Geometry: final body of the model. Coordinates: model frame, mm. A direction names the side the tool comes from. Give positions to 0.01 mm unless a question says otherwise; leave off trailing zeros. Write each loop counter-clockwise with the first axis right and the second up, starting at its lowest first coordinate (ties: lowest second). Pieces come first, ordered by that corner, then holes. Notation, with made-up numbers: M 8,49 L 33,49 A32 ccw 33,85 Z; hole C -17,39.25 d2. An arc over 180 degrees is marked long. Use one line per item in the form item = value. Start each with the question number.
Item 1: Section query A-A on z = -45.5. Return loops of the section in (x, y).
Item 2: Section query B-B on z = 90. Return loops of the section in (x, y), then the cut area to 3 significant figures.
Item 3: Contact query for flat-ended pins moving along their axis: P1, Ø1, axis at x = 14, y = -5, coming from the -Z side; P2, Ø4, axis at y = 7.5, z = 28.5, coming from the +X side; P3, Ø2.5, axis at x = -8.5, z = 10, coming from the +Y side; P4, Ø1.5, axis at x = -5.5, y = -1, coming from the +Z side. Output: stop coordinate, or through.
Item 4: Section query C-C on x = 3.75. Return loops of the section in (y, z), then the cut area to 3 significant figures.
Item 5: Pull-direction query (X, two-part tool) for faces 5 (the flat face through (8, 5.85, -1)), 6 (the flat face through (-9.1, 3, -93)), 7 (the flat face through (11, -2, 1)); classes: released by +X, released by -X, zero draft, split by the parting line, or undercut.
Item 6: Material intervals for line 1 along Y through (x, z) = (-0.5, 90); line 2 along X through (y, z) = (0, -89.5); line 3 along X through (y, z) = (8, -82.5), sorted ascending. Write a range as from..to.
Item 7: Access query for faces 1 (the flat face through (-9.1, 3, 94)), 2 (the cylindrical face through (7.217, 10.962, -97.535)), 3 (the flat face through (9.1, 3, 94)), 4 (the cylindrical face through (8.34, 2.87, 80.55)). Directions: +Z, -Z, +X, -X, +Y, -Y. A direction counts if a zero-diameter tool reaches every point of the face in a straight line with its end or side. Return the directions, or none.
Autodesk Inventor part; units mm, degrees
ref_plane "YZ Plane" through (0, 0, 0) normal (1, 0, 0) x (0, 1, 0)
ref_plane "XZ Plane" through (0, 0, 0) normal (0, 1, 0) x (-1, 0, 0)
ref_plane "XY Plane" through (0, 0, 0) normal (0, 0, 1) x (1, 0, 0)
sketch "Sketch1" plane through (0, 0, 0) normal (0, 0, 1) x (1, 0, 0)
  line L0 (-11, -8.3) -> (11, -8.3)
  line L1 (11, -8.3) -> (11, 8.3)
  line L2 (11, 8.3) -> (-11, 8.3)
  line L3 (-11, 8.3) -> (-11, -8.3)
  line L4 (-11, -8.3) -> (11, 8.3) construction
  line L5 (11, -8.3) -> (-11, 8.3) construction
  line L6 (-5.6, 8.3) -> (-5.6, 5.8)
  line L7 (-5.6, 5.8) -> (-9.1, 5.8)
  line L8 (-9.1, 5.8) -> (-9.1, -0.2)
  line L9 (-9.1, -0.2) -> (-5.6, -0.2)
  line L10 (-5.6, -0.2) -> (-5.6, -3.2)
  line L11 (-5.6, -3.2) -> (0, -3.2)
  line L12 (0, 8.3) -> (0, -8.3) construction
  line L13 (5.6, 8.3) -> (5.6, 5.8)
  line L14 (5.6, 5.8) -> (9.1, 5.8)
  line L15 (9.1, 5.8) -> (9.1, -0.2)
  line L16 (9.1, -0.2) -> (5.6, -0.2)
  line L17 (5.6, -0.2) -> (5.6, -3.2)
  line L18 (5.6, -3.2) -> (0, -3.2)
  point P0 (0, 0)
  point P1 (-5.6, 7.05)
  point P2 (-5.6, -1.7)
  point P3 (5.6, 8.3)
  dimension "d0" = 22
  dimension "d1" = 16.6
  dimension "d3" = 5.6
  dimension "d4" = 2.5
  dimension "d5" = 6
  dimension "d6" = 3
  dimension "d7" = 3.5
  dimension "d36" = 18.2
extrude "Extrusion1" add sketch "Sketch1" along normal mid plane 200 contours L3 L2 L6 L7 L8 L9 L10 L11 L18 L17 L16 L15 L14 L13 L1 L0
sketch "Sketch2" plane through (11, -8.3, 100) normal (1, 0, 0) x (0, 0, -1)
  line L0 (200, 16.6) -> (200, 0)
  line L1 (200, 0) -> (0, 0)
  circle A0 centre (190, 3) radius 1.65
  line L2 (0, 0) -> (0, 16.6)
  line L3 (200, 16.6) -> (0, 16.6)
  line L4 (100, 16.6) -> (100, 0)
  circle A1 centre (10, 3) radius 1.65
  point P0 (100, 8.3)
  dimension "d13" = 3.3
  dimension "d18" = 180
  dimension "d19" = 3
extrude "Extrusion2" cut sketch "Sketch2" against normal blind 180 contours A0 | A1
sketch "Sketch5" plane through (-11, -8.3, 100) normal (-1, 0, 0) x (0, 0, 1)
  line L0 (-185, 11.1) -> (-15, 11.1) construction
  line L1 (-185, 8.05) -> (-15, 8.05)
  line L2 (-15, 14.15) -> (-185, 14.15)
  arc A0 (-185, 14.15) -> (-185, 8.05) centre (-185, 11.1) ccw
  arc A1 (-15, 8.05) -> (-15, 14.15) centre (-15, 11.1) ccw
  line L3 (-200, 14.1) -> (-200, 8.1)
  line L4 (-200, 0) -> (0, 0)
  line L5 (-200, 16.6) -> (0, 16.6)
  line L6 (-100, 16.6) -> (-100, 8.05)
  point P0 (-100, 8.3)
  point P1 (-100, 11.1)
  point P2 (-200, 11.1)
  point P3 (-100, 0)
  dimension "d23" = 85
  dimension "d24" = 6.1
extrude "Extrusion4" cut sketch "Sketch5" against normal up to next
sketch "Sketch6" plane through (0, 0, 100) normal (0, 0, 1) x (1, 0, 0)
  line L0 (-11, 8.3) -> (-5.6, 8.3)
  arc A0 (-6.6, 8.3) -> (-9.8, 9.9) centre (-8.6, 8.3) ccw
  line L1 (-5.6, 8.3) -> (-11, 8.3)
  arc A1 (-5.6, 8.3) -> (-10.4, 10.7) centre (-8.6, 8.3) ccw
  arc A2 (-10.4, 10.7) -> (-9.8, 9.9) centre (-10.1, 10.3) ccw
  line L2 (-11, 8.3) -> (-11, -8.3)
  point P0 (0, 0)
  point P1 (-6.5, 8.3)
  dimension "d29" = 2
  dimension "d31" = 1
  dimension "d32" = 2
extrude "Extrusion5" add sketch "Sketch6" against normal blind 5
mirror "Mirror1" about plane through (0, 0, 0) normal (1, 0, 0) of "Extrusion5"
mirror "Mirror2" about plane through (0, 0, 0) normal (0, 0, 1) of "Extrusion5", "Mirror1"
mirror "Mirror3" about plane through (0, 0, 0) normal (1, 0, 0) of "Extrusion4"
sketch "Sketch7" plane through (11, -8.3, 100) normal (1, 0, 0) x (0, 0, -1)
  line L0 (170, 11.1) -> (185, 11.1) construction
  line L1 (170, 8.05) -> (185, 8.05)
  line L2 (185, 14.15) -> (170, 14.15)
  arc A0 (170, 14.15) -> (170, 8.05) centre (170, 11.1) ccw
  arc A1 (185, 8.05) -> (185, 14.15) centre (185, 11.1) ccw
  arc A2 (185, 8.05) -> (185, 14.15) centre (185, 11.1) ccw
  arc A3 (177.5, 8.05) -> (177.5, 14.15) centre (177.5, 11.1) ccw
  point P0 (100, 8.3)
  dimension "d37" = 15
extrude "Extrusion6" add sketch "Sketch7" against normal up to surface (5.4 mm away) contours A3 L2 A1 L1
sketch "Sketch8" plane through (11, -8.3, 100) normal (1, 0, 0) x (0, 0, -1)
  circle A0 centre (182, 10.6) radius 0.95
  circle A1 centre (182, 3.6) radius 1.05
  line L0 (181.05, 4.0472) -> (181.05, 3.1528)
  line L1 (182, 4.65) -> (182, 2.55)
  line L2 (182.95, 4.0472) -> (182.95, 3.1528)
  line L3 (0, 16.6) -> (200, 16.6)
  line L4 (200, 16.6) -> (200, 0)
  point P0 (100, 8.3)
  point P1 (182.95, 3.1528)
  point P2 (182.95, 4.0472)
  dimension "d40" = 1.9
  dimension "d41" = 2.1
  dimension "d42" = 1.9
  dimension "d43" = 7
  dimension "d44" = 6
  dimension "d45" = 18
extrude "Extrusion7" add sketch "Sketch8" along normal blind 6.2 contours A0 | L2 A1 L1 | L1 A1 L0
mirror "Mirror4" about plane through (0, 0, 0) normal (0, 0, 1) of "Extrusion6", "Extrusion7"
ref_plane "Work Plane1" through (0, 0, 0) normal (1, 0, 0) x (0, 1, 0)
ref_plane "Work Plane2" through (0, 0, 0) normal (-1, 0, 0) x (0, 1, 0)
ref_plane "Work Plane3" through (0, 0, 0) normal (-1, 0, 0) x (0, 1, 0)
equation "\"d15\" = d18"
properties part number "Rack ( Female Fixation )"
Answer sheet:
q1.outline = M -11,-8.3 L 11,-8.3 L 11,-0.25 L 5.6,-0.25 L 5.6,-3.2 L -5.6,-3.2 L -5.6,-0.25 L -11,-0.25 Z; M -11,5.85 L -5.6,5.85 L -5.6,8.3 L -11,8.3 Z; M 5.6,5.85 L 11,5.85 L 11,8.3 L 5.6,8.3 Z
q2.outline = M -11,-8.3 L 11,-8.3 L 11,-6.95 L -11,-6.95 Z; M -11,-3.65 L 11,-3.65 L 11,8.3 L 5.6,8.3 L 5.6,5.8 L 9.1,5.8 L 9.1,-0.2 L 5.6,-0.2 L 5.6,-3.2 L -5.6,-3.2 L -5.6,-0.2 L -9.1,-0.2 L -9.1,5.8 L -5.6,5.8 L -5.6,8.3 L -11,8.3 Z
q2.area = 122 mm2
q3.P1 = -82.95
q3.P2 = 11
q3.P3 = 8.3
q3.P4 = 100
q4.outline = M -8.3,-100 L -3.2,-100 L -3.2,100 L -8.3,100 Z; hole C -5.3,-90 d3.3; hole C -5.3,90 d3.3
q4.area = 1,000 mm2
q5.face_5 = zero draft
q5.face_6 = undercut
q5.face_7 = released by +X
q6.line_1 = -8.3..-6.95, -3.65..-3.2
q6.line_2 = -11..-9.1, 9.1..11
q6.line_3 = -11..-5.6, 5.6..11
q7.face_1 = +Z, -Z
q7.face_2 = +Z, -Z, +Y
q7.face_3 = +Z
q7.face_4 = +X, -X
